Could you check a few things on this model? Use its own coordinates, in mm. Give positions to 0.01 mm unless a question says otherwise; leave off trailing zeros. Loops run counter-clockwise (first coordinate to the right, second up) from the corner with the lowest first, then second, coordinate; pieces in that order, holes last. Notation, with made-up numbers: (40.25, -34.75) - (99.25, -34.75) arc R25 cw to (99.25, -12.75) - close; hole circle Ø5 at (73, -2). An arc over 180 degrees is marked (long way). Use CSV: the item, a comma, the result in double quotes.
from build123d import *

# Parameters (mm, degrees)
F0_R     = 0.25
F1_DEPTH = 0.5


with BuildPart() as f1:
    # F0 (on Top) → F1 (new body)
    with BuildSketch(Plane.XY):
        with BuildLine():
            Line((0.75, -4), (0.75, 4))
            ThreePointArc((0.75, 4), (0.53033, 4.53033), (0, 4.75))
            ThreePointArc((0, 4.75), (-0.53033, 4.53033), (-0.75, 4))
            Line((-0.75, 4), (-0.75, -4))
            ThreePointArc((-0.75, -4), (-0.53033, -4.53033), (0, -4.75))
            ThreePointArc((0, -4.75), (0.53033, -4.53033), (0.75, -4))
        make_face()
        with Locations((0, -4)):
            Circle(F0_R, mode=Mode.SUBTRACT)
        with Locations((0, 4)):
            Circle(F0_R, mode=Mode.SUBTRACT)
    extrude(amount=F1_DEPTH)


solid = f1.part
1) Suppose I cut it at B-B (x = 0.5). Please give me the cut outline in (y, z), plus the area to 3 significant figures.
Answer below:
outline,"(-4.56, 0) - (4.56, 0) - (4.56, 0.5) - (-4.56, 0.5) - close"
area,"4.56 mm2"
2) Suppose I cut it at A-A (z = 0.2). Please give me the cut outline in (x, y), plus the area to 3 significant figures.
Answer below:
outline,"(-0.75, -4) arc R0.75 ccw to (0.75, -4) - (0.75, 4) arc R0.75 ccw to (-0.75, 4) - close; hole circle Ø0.5 at (0, -4); hole circle Ø0.5 at (0, 4)"
area,"13.4 mm2"
3) I need wall thicknesses on line 1 along Y through (x, z) = (0.1, 0.15); line 2 along Y through (x, z) = (0.35, 0.1); line 3 along Y through (x, z) = (-0.45, 0.35). Which ranges of each line are inside material? Lowest first, please.
Answer below:
line 1,"y = -4.74 to -4.23, -3.77 to 3.77, 4.23 to 4.74"
line 2,"y = -4.66 to 4.66"
line 3,"y = -4.6 to 4.6"
